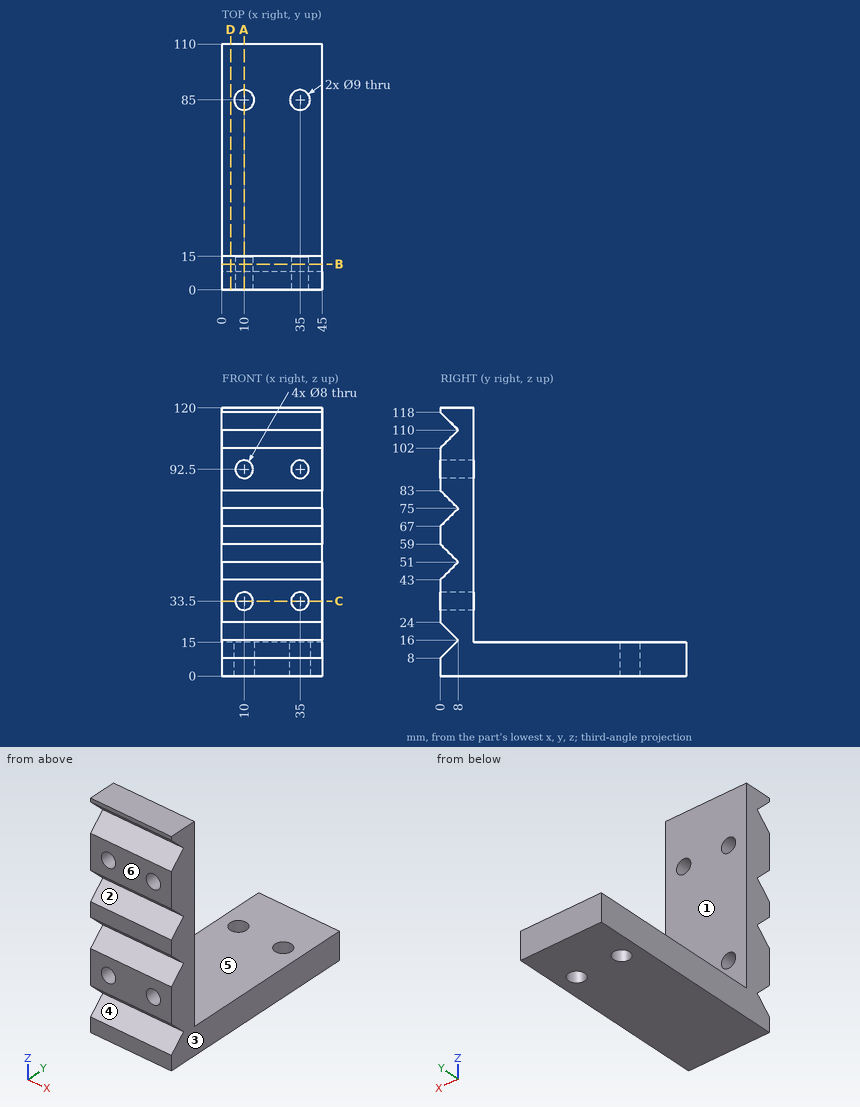
The figure shows three views and two pictorial views of one solid part (mm, origin at its lowest corner). Answer the questions. A direction names the side the tool comes from. Round coordinates to 2 decimals unless told otherwise and drop trailing zeros. Write each loop counter-clockwise with the first axis right and the second up, starting at its lowest first coordinate (ties: lowest second). Pieces come first, ordered by that corner, then holes. Notation, with made-up numbers: (31, -4) -> (78, -4) arc R11 ccw to (78, 8) -> close; hole circle Ø4 at (28.5, 88.5). An arc over 180 degrees is marked (long way). Answer as a JSON object with one key per item and string values. Group by question number.
Q1. Straight lines are drawn through the part: line 1 along X through (y, z) = (8, 92); line 2 along Z through (x, y) = (10, 9.5); line 3 along Z through (x, y) = (26.5, 26). For each, find the intervals that lie inside material, in ascending order.
Q2. Section A-A (x = 10) is taken. Count the separate pieces of the cut face and the enclosed holes in it, plus the area to 3 significant figures.
Q3. Section B-B (y = 11.5) is taken. Write down the section's boundary in (x, z), plus the area to 3 significant figures.
Q4. Each of these flat-tipped pins is pushed along its axis until it touches: pin 1 Ø6.5 at (x, z) = (10, 33.5) entering from -Y; pin 2 Ø4 at (x, z) = (27.5, 85.5) entering from +Y; pin 3 Ø12 at (x, y) = (26, 71) entering from +Z; pin 4 Ø4 at (x, z) = (36.5, 48) entering from -Y. Where does it stop, or does it pass through?
Q5. Which of the six approach directions +Z, -Z, +X, -X, +Y, -Y give full straight-line access (tool end or side, diameter ignored) to the marked faces 1, 2 and 3?
Q6. Determine the mould class of the marked faces 4, 5 and 6 for opening direction Z: pulls with the +Z half, pulls with the -Z half, needs draft (parallel to the pull), parting line crosses it, or undercut.
Q7. Section D-D (x = 4) is taken. Write down the section's boundary in (y, z).
Q8. Section C-C (z = 33.5) is taken. Write down the section's boundary in (x, y).
Check values:
{
 "1": {"line 1": "0 to 6.03, 13.97 to 31.03, 38.97 to 45", "line 2": "0 to 29.5, 37.5 to 88.5, 96.5 to 120", "line 3": "0 to 15"},
 "2": {"separate pieces": "4", "enclosed holes": "0", "area": "2,590 mm^2"},
 "3": {"outline": "(0, 0) -> (45, 0) -> (45, 120) -> (0, 120) -> close; hole circle Ø8 at (10, 33.5); hole circle Ø8 at (10, 92.5); hole circle Ø8 at (35, 33.5); hole circle Ø8 at (35, 92.5)", "area": "5,200 mm^2"},
 "4": {"pin 1": "through", "pin 2": "y = 15", "pin 3": "z = 15", "pin 4": "y = 3"},
 "5": {"face 1": "+Z, +X, -X, +Y", "face 2": "+X, -X, -Y", "face 3": "+Z, -Z, +X, +Y, -Y"},
 "6": {"face 4": "undercut", "face 5": "pulls with the +Z half", "face 6": "needs draft"},
 "7": {"outline": "(0, 0) -> (110, 0) -> (110, 15) -> (15, 15) -> (15, 120) -> (0, 120) -> (0, 118) -> (8, 110) -> (0, 102) -> (0, 83) -> (8, 75) -> (0, 67) -> (0, 59) -> (8, 51) -> (0, 43) -> (0, 24) -> (8, 16) -> (0, 8) -> close"},
 "8": {"outline": "(0, 0) -> (6, 0) -> (6, 15) -> (0, 15) -> close; (14, 0) -> (31, 0) -> (31, 15) -> (14, 15) -> close; (39, 0) -> (45, 0) -> (45, 15) -> (39, 15) -> close"}
}
